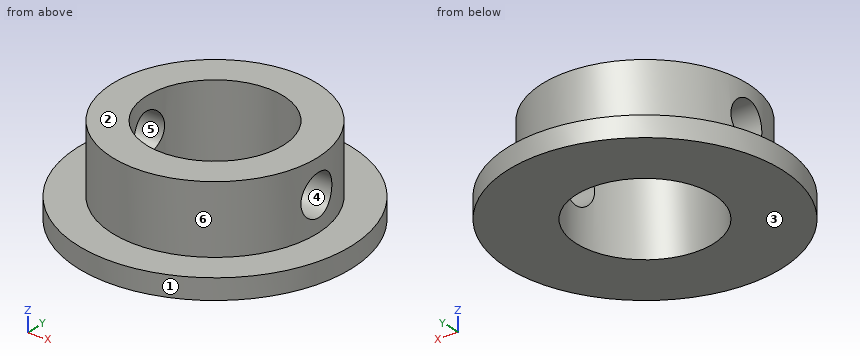
from build123d import *

# Parameters (mm, degrees)
SKETCH_1_R          = 10
EXTRUDE_1_DEPTH     = 1.5
SKETCH_2_R          = 7.5
EXTRUDE_2_DEPTH     = 5
SKETCH_3_R          = 5
CUT_EXTRUDE_1_DEPTH = 16.564382416
SKETCH_4_R          = 1.5
CUT_EXTRUDE_2_DEPTH = 22.177818585


with BuildPart() as part:
    # 草图1 → 凸台-拉伸1 (new body)
    with BuildSketch(Plane.XY):
        Circle(SKETCH_1_R)
    extrude(amount=EXTRUDE_1_DEPTH)

    # 草图2 → 凸台-拉伸2 (add)
    with BuildSketch(Plane.XY.offset(1.5)):
        Circle(SKETCH_2_R)
    extrude(amount=EXTRUDE_2_DEPTH)

    # 草图3 → 切除-拉伸1 (cut, through all)
    with BuildSketch(Plane.XY.offset(6.5)):
        Circle(SKETCH_3_R)
    extrude(amount=-CUT_EXTRUDE_1_DEPTH, mode=Mode.SUBTRACT)

    # 草图4 → 切除-拉伸2 (cut, through all)
    with BuildSketch(Plane(origin=(7.5, 0, 0), x_dir=(0, 0, -1), z_dir=(1, 0, 0))):
        with Locations((-4, 0)):
            Circle(SKETCH_4_R)
    extrude(amount=-CUT_EXTRUDE_2_DEPTH, mode=Mode.SUBTRACT)


solid = part.part
Can you work these out from the model? Positions are in its coordinate system, mm. Face numbers are marked on the shaded views. A direction names the side the tool comes from. Round coordinates to 2 decimals unless told otherwise and drop trailing zeros. Order: outer loops, then holes, each group sorted by start corner. A loop starts at its lowest first (then second) coordinate and runs counter-clockwise, first axis right, second up. Notation, with made-up numbers: (80, -38) -> (85, -38) arc R22 cw to (85, -20) -> close; hole circle Ø5 at (81, -22.75). An arc over 180 degrees is marked (long way). Write each question's results on one line, items separated by ' | '. Start each with the question number.
Item 1: Please list where these lines run through material, in increasing order: L1, parallel to Z at x = 7.25, y = 0; L2, parallel to Y at x = 0, z = 2.5; L3, parallel to Y at x = 6.75, z = 4.5.
Item 2: If we section it at C-C, the plane z = 4.75: Write out the boundary of the cut face in (x, y), then the cut area to 3 significant figures.
Item 3: If we section it at D-D, the plane y = 2: Write out the boundary of the cut face in (x, z).
Item 4: If we section it at B-B, the plane y = 0: Write out the boundary of the cut face in (x, z), then the cut area to 3 significant figures.
Item 5: Which directions (+Z, -Z, +X, -X, +Y, -Y) give clear straight access to the entire face, cutting with the end or side of a thin tool? Please do the marked faces 5 and 6.
Item 6: Thinking about a two-plate mould opening in Z: for the marked faces 1, 2, 3 and 4, which applies, +Z half, -Z half, draft (parallel to the pull), parting line (faces both ways), or undercut?
Item 7: Will these pins go through, and if not, where does the flat tip stop? pin 1 (3.5 mm diameter, centred on y = 0, z = 4, fed in from +X); pin 2 (1 mm diameter, centred on y = -4, z = 0.5, fed in from +X); pin 3 (2 mm diameter, centred on x = -2, z = 3.5, fed in from +Y).
Item 8: If we section it at A-A, the plane x = 0: Write out the boundary of the cut face in (y, z).
Results:
1) L1: z = 0 to 2.5, 5.5 to 6.5 | L2: y = -7.5 to -5, 5 to 7.5 | L3: y = -3.27 to -1.41, 1.41 to 3.27
2) outline: (-7.39, -1.3) arc R7.5 ccw to (7.39, -1.3) -> (4.83, -1.3) arc R5 cw to (-4.83, -1.3) -> close; (-7.39, 1.3) -> (-4.83, 1.3) arc R5 cw to (4.83, 1.3) -> (7.39, 1.3) arc R7.5 ccw to start | area: 85.1 mm2
3) outline: (-9.8, 0) -> (-4.58, 0) -> (-4.58, 6.5) -> (-7.23, 6.5) -> (-7.23, 1.5) -> (-9.8, 1.5) -> close; (4.58, 0) -> (9.8, 0) -> (9.8, 1.5) -> (7.23, 1.5) -> (7.23, 6.5) -> (4.58, 6.5) -> close
4) outline: (-10, 0) -> (-5, 0) -> (-5, 2.5) -> (-7.5, 2.5) -> (-7.5, 1.5) -> (-10, 1.5) -> close; (-7.5, 5.5) -> (-5, 5.5) -> (-5, 6.5) -> (-7.5, 6.5) -> close; (5, 0) -> (10, 0) -> (10, 1.5) -> (7.5, 1.5) -> (7.5, 2.5) -> (5, 2.5) -> close; (5, 5.5) -> (7.5, 5.5) -> (7.5, 6.5) -> (5, 6.5) -> close | area: 25.0 mm2
5) face 5: +X, -X | face 6: +Z
6) face 1: draft | face 2: +Z half | face 3: -Z half | face 4: undercut
7) pin 1: stops at x = 7.5 | pin 2: stops at x = 9.37 | pin 3: stops at y = 7.43
8) outline: (-10, 0) -> (-5, 0) -> (-5, 6.5) -> (-7.5, 6.5) -> (-7.5, 1.5) -> (-10, 1.5) -> close; (5, 0) -> (10, 0) -> (10, 1.5) -> (7.5, 1.5) -> (7.5, 6.5) -> (5, 6.5) -> close
